```python
from build123d import *

# Parameters (mm, degrees)
BOSS_EXTRUDE1_DEPTH       = 3.175
SKETCH3_R                 = 3.048
CUT_FOR_AXLE_DEPTH        = 4.175
SKETCH4_W                 = 6.35
SKETCH4_H                 = 3.2258
CUT_FOR_TABS_DEPTH        = 4.175
CUT_FOR_CLEARANCE_DEPTH   = 4.175
CUT_EXTRUDE1_DEPTH        = 4.175
SKETCH10_W                = 3.2258
SKETCH10_H                = 6.35
TABS_FOR_BACK_PLATE_DEPTH = 3.175


with BuildPart() as part:
    # Sketch1 → Boss-Extrude1 (new body)
    with BuildSketch(Plane(origin=(0, 0, 0), x_dir=(0, 0, -1), z_dir=(1, 0, 0))):
        with BuildLine():
            Line((-8.901335672, 27.917328656), (29.198664328, 27.917328656))
            Line((29.198664328, 27.917328656), (52.058664328, 27.917328656))
            ThreePointArc((52.058664328, 27.917328656), (54.100437174, 20.297328656), (52.058664328, 12.677328656))
            Line((52.058664328, 12.677328656), (29.198664328, -0.520898498))
            Line((29.198664328, -0.520898498), (29.198664328, -54.632671344))
            Line((29.198664328, -54.632671344), (-8.901335672, -54.632671344))
            Line((-8.901335672, -54.632671344), (-8.901335672, 27.917328656))
        make_face()
    extrude(amount=BOSS_EXTRUDE1_DEPTH)

    # Sketch3 → cut for axle (cut, through all)
    with BuildSketch(Plane(origin=(3.175, 0, 0), x_dir=(0, 0, -1), z_dir=(1, 0, 0))):
        with Locations((46.978664328, 20.297328656)):
            Circle(SKETCH3_R)
    extrude(amount=-CUT_FOR_AXLE_DEPTH, mode=Mode.SUBTRACT)

    # Sketch4 → cut for tabs (cut, through all)
    with BuildSketch(Plane(origin=(3.175, 0, 0), x_dir=(0, 0, -1), z_dir=(1, 0, 0))):
        with Locations((0.623664328, -49.971771344)):
            Rectangle(SKETCH4_W, SKETCH4_H)
        with Locations((19.673664328, -49.971771344)):
            Rectangle(SKETCH4_W, SKETCH4_H)
        Polygon((10.148664328, -54.632671344), (6.973664328, -54.632671344), (6.973664328, -51.457671344), (13.323664328, -51.457671344), (13.323664328, -54.632671344), align=None)
    extrude(amount=-CUT_FOR_TABS_DEPTH, mode=Mode.SUBTRACT)

    # Sketch6 → cut for clearance (cut, through all)
    with BuildSketch(Plane(origin=(3.175, 0, 0), x_dir=(0, 0, -1), z_dir=(1, 0, 0))):
        Polygon((29.198664328, -0.520898498), (21.256966839, -24.543474446), (29.198664328, -27.939523247), align=None)
    extrude(amount=-CUT_FOR_CLEARANCE_DEPTH, mode=Mode.SUBTRACT)

    # Sketch9 → Cut-Extrude1 (cut, through all)
    with BuildSketch(Plane.ZY):
        Polygon((8.901335672, 27.917328656), (-29.198664328, 27.917328656), (8.901335672, 15.979328656), align=None)
    extrude(amount=-CUT_EXTRUDE1_DEPTH, mode=Mode.SUBTRACT)

    # Sketch10 → tabs for back plate (add)
    with BuildSketch(Plane.ZY):
        with Locations((10.514235672, -6.245671344)):
            Rectangle(SKETCH10_W, SKETCH10_H)
        with Locations((10.514235672, -18.945671344)):
            Rectangle(SKETCH10_W, SKETCH10_H)
    extrude(amount=-TABS_FOR_BACK_PLATE_DEPTH)


solid = part.part
```
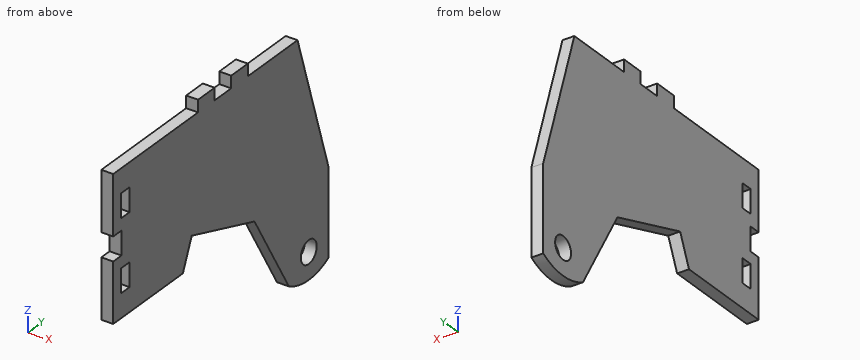
Design review of the part built by this model. Coordinates are the model's own, in mm. Round coordinates to 2 decimals unless told otherwise and drop trailing zeros. Write each loop counter-clockwise with the first axis right and the second up, starting at its lowest first coordinate (ties: lowest second). Pieces come first, ordered by that corner, then holes.
Item 1: We need section B-B on x = 1.9. State how many separate pieces and enclosed holes the cut face has, and give its area (3 significant figures).
Item 2: For probe 1 along Z at (x, y) = (1.25, -40); probe 2 along Y at (x, z) = (1.6, -45); probe 3 along Y at (x, z) = (1.4, -1.5), list the stretches that pass through material, from the lowest coordinate up.
Item 3: We need section D-D on z = -24.5. Write out the cut boundary in (x, y) (3 decimals), and give its area (3 significant figures).
Item 4: Clearance check with flat-ended pins moving along their axes: pin 1 Ø1 at (x, y) = (1, -9.5) entering from -Z; pin 2 Ø1 at (x, y) = (2, -12) entering from +Z. State where each tip first meets the part, or that it passes through.
Item 5: We need section C-C on y = -36. Write out the cut boundary in (x, z) (3 decimals).
Item 6: We need section A-A on z = 0. Write out the cut boundary in (x, y) (3 decimals), and give its area (3 significant figures).
Returned:
1. separate pieces: 1
1. enclosed holes: 3
1. area: 3,280 mm2
2. probe 1: z = -29.2 to 8.9
2. probe 2: y = 8.6 to 17.98, 22.62 to 27.92
2. probe 3: y = -54.63 to -51.58, -48.36 to 19.24
3. outline: (0, -54.633) - (3.175, -54.633) - (3.175, -25.93) - (0, -25.93) - close; (0, -14.734) - (3.175, -14.734) - (3.175, 26.445) - (0, 26.445) - close
3. area: 222 mm2
4. pin 1: stops at z = -26.4
4. pin 2: stops at z = 8.9
5. outline: (0, -29.199) - (3.175, -29.199) - (3.175, 8.901) - (0, 8.901) - close
6. outline: (0, -54.633) - (3.175, -54.633) - (3.175, -51.585) - (0, -51.585) - close; (0, -48.359) - (3.175, -48.359) - (3.175, 18.768) - (0, 18.768) - close
6. area: 223 mm2
